Source: CAD feature listing. Evaluate the final solid. Frame: model axes, mm. A direction names the side the tool comes from. Give positions to 0.01 mm unless a question says otherwise; leave off trailing zeros. Loops run counter-clockwise (first coordinate to the right, second up) from the corner with the lowest first, then second, coordinate; pieces in that order, holes last. Notation, with made-up numbers: M 28.25,18.25 L 56.25,18.25 A20 cw 56.25,28.25 Z; hole C 38,45.25 d5. An arc over 180 degrees is marked long. Put each result on its own line as item: value.
from build123d import *

# Parameters (mm, degrees)
CUT_EXTRUDE1_DEPTH      = 216.9
CUT_EXTRUDE1_DEPTH_BACK = 216.9
SKETCH4_R               = 50.8
BOSS_EXTRUDE1_DEPTH     = 25.4


with BuildPart() as part:
    # Sketch2 → Revolve1 (revolve)
    with BuildSketch(Plane.XY):
        with BuildLine():
            Line((0, 0), (215.9, 0))
            Line((215.9, 0), (215.9, -304.8))
            ThreePointArc((215.9, -304.8), (152.664354058, -457.464354058), (0, -520.7))
            Line((0, -520.7), (0, 0))
        make_face()
    revolve(axis=Axis((0, 0, 0), (0, -1, 0)))

    # Sketch3 → Cut-Extrude1 (cut, two sides)
    with BuildSketch(Plane.XY) as cut_extrude1_sk:
        with BuildLine():
            Line((190.5, -215.9), (190.5, -546.1))
            Line((190.5, -546.1), (-190.5, -546.1))
            Line((-190.5, -546.1), (-190.5, -215.9))
            ThreePointArc((-190.5, -215.9), (0, -94.577593963), (190.5, -215.9))
        make_face()
    extrude(amount=CUT_EXTRUDE1_DEPTH, mode=Mode.SUBTRACT)
    extrude(cut_extrude1_sk.sketch, amount=-CUT_EXTRUDE1_DEPTH_BACK, mode=Mode.SUBTRACT)

    # Sketch4 → Boss-Extrude1 (add)
    with BuildSketch(Plane(origin=(-190.5, 0, 0), x_dir=(0, 0, -1), z_dir=(1, 0, 0))):
        with Locations((0, -311.15)):
            Circle(SKETCH4_R)
    boss_extrude1 = extrude(amount=BOSS_EXTRUDE1_DEPTH)

    # Mirror1: Boss-Extrude1 across plane
    add(boss_extrude1.mirror(Plane(origin=(0, 0, 0), x_dir=(0, 0, 1), z_dir=(1, 0, 0))))


solid = part.part
1. Access query for faces 1 (the cylindrical face through (205.93, -120.67, 64.85)), 2 (the cylindrical face through (-177.978, -360.742, 11.012)), 3 (the flat face through (165.1, -310, 1)). Directions: +Z, -Z, +X, -X, +Y, -Y. A direction counts if a zero-diameter tool reaches every point of the face in a straight line with its end or side. Return the directions, or none.
Found:
face 1: +Y, -Y
face 2: none
face 3: +Z, -Z, -Y
2. Section query B-B (y = -311.15). Output: boundary loops of the cut face in (x, z).
Found:
outline: M -190.5,-101.4 L -190.5,-50.8 L -165.1,-50.8 L -165.1,50.8 L -190.5,50.8 L -190.5,101.4 A215.81 ccw Z; M 165.1,-50.8 L 190.5,-50.8 L 190.5,-101.4 A215.81 ccw 190.5,101.4 L 190.5,50.8 L 165.1,50.8 Z
3. Section query C-C (x = 0). Output: boundary loops of the cut face in (y, z).
Found:
outline: M -94.58,-215.9 L 0,-215.9 L 0,215.9 L -94.58,215.9 Z
4. Draft query along Y for faces 4 (the flat face through (3, 0, 3)), 5 (the cylindrical face through (177.978, -360.742, 11.012)), 6 (the flat face through (190.5, -289, -47)), 7 (the flat face through (-165.1, -310, 1)). Return one class per face: pulls with the +Y half, pulls with the -Y half, needs draft (parallel to the pull), parting line crosses it, or undercut.
Found:
face 4: pulls with the +Y half
face 5: undercut
face 6: undercut
face 7: needs draft
5. Contact query for flat-ended pins moving along their axis: P1, Ø5, axis at x = -30.5, z = 73.5, coming from the +Y side; P2, Ø10, axis at x = 120, y = -101, coming from the +Z side; P3, Ø10, axis at x = -101.5, y = -92.5, coming from the -Z side; P4, Ø3, axis at x = -78.5, z = 39.5, coming from the -Y side. Output: stop coordinate, or through.
Found:
P1: y = 0
P2: z = 182.72
P3: z = -193.13
P4: y = -110.39
6. Section query A-A (z = 0). Output: boundary loops of the cut face in (x, y), plus the area to 3 significant figures.
Found:
outline: M -215.9,-304.8 A215.9 ccw -190.5,-406.4 L -190.5,-361.95 L -165.1,-361.95 L -165.1,-260.35 L -190.5,-260.35 L -190.5,-215.9 A210.22 cw 190.5,-215.9 L 190.5,-260.35 L 165.1,-260.35 L 165.1,-361.95 L 190.5,-361.95 L 190.5,-406.4 A215.9 ccw 215.9,-304.8 L 215.9,0 L -215.9,0 Z
area: 73,200 mm^2
7. Material intervals for line 1 (X direction, y = -293, z = 12); line 2 (X direction, y = -123.5, z = 105.5); line 3 (Y direction, x = 2.5, z = -40), sorted ascending. Write a range as from..to.
Found:
line 1: -215.57..-165.1, 165.1..215.57
line 2: -188.37..-106.41, 106.41..188.37
line 3: -94.59..0
8. Section query D-D (y = -60). Output: boundary loops of the cut face in (x, z), plus the area to 3 significant figures.
Found:
outline: C 0,0 d431.8
area: 146,000 mm^2
